Could you check a few things on this model? Use its own coordinates, in mm. A direction names the side the tool comes from. Coordinates: 2 decimals unless noted, no trailing zeros. Loops run counter-clockwise (first coordinate to the right, second up) from the corner with the lowest first, then second, coordinate; pieces in that order, holes last.
1) Thinking about a two-plate mould opening in X: for faces 3 (the face through (-0.35, 5.44, 1.97)), 4 (the face through (4.715, 9.699, 2.028)), 5 (the face through (-0.35, -8.56, 1.97)), 6 (the face through (-2.715, -9.699, 2.028)), which applies, released by +X, released by -X, zero draft, split by the parting line, or undercut?
2) Imagine slicing it at A-A on z = 0.3. Please give me the cut outline in (x, y).
3) Imagine slicing it at B-B on x = 0. Please give me the cut outline in (y, z), plus the area to 4 significant figures.
4) Imagine slicing it at D-D on z = 1.85. Please give me the cut outline in (x, y), plus the area to 3 significant figures.
5) For faces 1 (the face through (5, 0, 2)), 2 (the face through (1, 0, 0.5)), which set-ups out of +Z, -Z, +X, -X, +Y, -Y let a thin tool reach every point of the face, with its end or its side?
6) Will this pin go through, and if not, where does the flat tip stop? P1, Ø2, axis at x = 1, y = -0.5, coming from the -Z side.
7) If I drill on line 1 along Y through (x, z) = (0, 2.4); line 2 along X through (y, z) = (-7, 3.1); line 3 along X through (y, z) = (-6.5, 3.8), over which ranges is the centre line in solid material (lowest first)?
8) Imagine slicing it at C-C on y = 7. Please give me the cut outline in (x, z).
```python
from build123d import *

# Parameters (mm, degrees)
BOX009_W          = 10
BOX009_H          = 6.5
BOX009_DEPTH      = 0.5
CYLINDER012_R     = 1.6
CYLINDER012_DEPTH = 10
CYLINDER011_R     = 1.6
CYLINDER011_DEPTH = 10
BOX008_W          = 8
BOX008_H          = 20
BOX008_DEPTH      = 4
FILLET002_R       = 1


with BuildPart() as cube009:
    # Box009 → Box009 (new body)
    with BuildSketch(Plane(origin=(-4, -3.25, 0), x_dir=(1, 0, 0), z_dir=(0, 0, 1))):
        with Locations((5, 3.25)):
            Rectangle(BOX009_W, BOX009_H)
    extrude(amount=BOX009_DEPTH)


with BuildPart() as cylinder012:
    # Cylinder012 → Cylinder012 (new body)
    with BuildSketch(Plane(origin=(0, -7, 0), x_dir=(1, 0, 0), z_dir=(0, 0, 1))):
        Circle(CYLINDER012_R)
    extrude(amount=CYLINDER012_DEPTH)


with BuildPart() as fusion017:
    # Cylinder011 → Cylinder011 (new body)
    with BuildSketch(Plane(origin=(0, 7, 0), x_dir=(1, 0, 0), z_dir=(0, 0, 1))):
        Circle(CYLINDER011_R)
    extrude(amount=CYLINDER011_DEPTH)

    # Fusion017: union Cylinder012
    add(cylinder012.part)


with BuildPart() as belt_clamp002:
    # Box008 → Box008 (new body)
    with BuildSketch(Plane(origin=(-3, -10, 0), x_dir=(1, 0, 0), z_dir=(0, 0, 1))):
        with Locations((4, 10)):
            Rectangle(BOX008_W, BOX008_H)
    extrude(amount=BOX008_DEPTH)

    # Fillet002
    fillet002_edges = [belt_clamp002.edges().sort_by_distance(p)[0] for p in [
        (-3, -10, 2),
        (-3, 10, 2),
        (5, -10, 2),
        (5, 10, 2),
    ]]
    fillet(fillet002_edges, radius=FILLET002_R)

    # Cut008004003012001003001009: cut Fusion017
    add(fusion017.part, mode=Mode.SUBTRACT)

    # Cut008004003012001003001010: cut Cube009
    add(cube009.part, mode=Mode.SUBTRACT)


solid = belt_clamp002.part
```
Filled in:
1. face 3: undercut
1. face 4: released by +X
1. face 5: undercut
1. face 6: released by -X
2. outline: (-3, -9) arc R1 ccw to (-2, -10) - (4, -10) arc R1 ccw to (5, -9) - (5, -3.25) - (-3, -3.25) - close; (-3, 3.25) - (5, 3.25) - (5, 9) arc R1 ccw to (4, 10) - (-2, 10) arc R1 ccw to (-3, 9) - close; hole circle Ø3.2 at (0, -7); hole circle Ø3.2 at (0, 7)
3. outline: (-10, 0) - (-8.6, 0) - (-8.6, 4) - (-10, 4) - close; (-5.4, 0) - (-3.25, 0) - (-3.25, 0.5) - (3.25, 0.5) - (3.25, 0) - (5.4, 0) - (5.4, 4) - (-5.4, 4) - close; (8.6, 0) - (10, 0) - (10, 4) - (8.6, 4) - close
3. area: 51.15 mm2
4. outline: (-3, -9) arc R1 ccw to (-2, -10) - (4, -10) arc R1 ccw to (5, -9) - (5, 9) arc R1 ccw to (4, 10) - (-2, 10) arc R1 ccw to (-3, 9) - close; hole circle Ø3.2 at (0, -7); hole circle Ø3.2 at (0, 7)
4. area: 143 mm2
5. face 1: +Z, -Z, +X, +Y, -Y
5. face 2: -Z, +X, -X
6. P1: stops at z = 0.5
7. line 1: y = -10 to -8.6, -5.4 to 5.4, 8.6 to 10
7. line 2: x = -3 to -1.6, 1.6 to 5
7. line 3: x = -3 to -1.52, 1.52 to 5
8. outline: (-3, 0) - (-1.6, 0) - (-1.6, 4) - (-3, 4) - close; (1.6, 0) - (5, 0) - (5, 4) - (1.6, 4) - close
